Work out the finished part from the listing and answer in its coordinate system (mm). A direction names the side the tool comes from. Coordinates: 2 decimals unless noted, no trailing zeros. Write each loop counter-clockwise with the first axis right and the second up, starting at its lowest first coordinate (ties: lowest second). Pieces come first, ordered by that corner, then holes. Notation, with made-up numbers: (-6.5, 84) - (17.5, 84) arc R29 cw to (17.5, 112) - close; hole circle Ø3 at (75, 37). An arc over 180 degrees is marked (long way). Use one line per item in the form item = value. Start each with the question number.
Item 1: A cutting plane is placed at B-B (x = -5.5). Write down the section's boundary in (y, z), then the cut area to 3 significant figures.
Item 2: A cutting plane is placed at C-C (z = 4). Write down the section's boundary in (x, y) (3 decimals).
Item 3: For faces 4 (the cylindrical face through (-3.971, -3.045, 0.739)), 5 (the flat face through (-4.7, 1.25, -11.6)), 6 (the flat face through (-5.1, 1, -12)), 7 (the flat face through (5.1, 1, -12)), 8 (the flat face through (0, -4.4, 0)), determine the directions among +Z, -Z, +X, -X, +Y, -Y from which every point of the face is accessible in a straight line to the end or side of a thin tool.
Item 4: A cutting plane is placed at A-A (z = -7). Write down the section's boundary in (x, y).
Item 5: Consider probe 1 along Z at (x, y) = (-1.25, 2); probe 2 along Z at (x, y) = (-5, -2.5); probe 3 along Y at (x, z) = (5.25, -7). Determine where each line is inside the solid, lowest interval first.
Item 6: Determine the mould class of faces 1 (the cylindrical face through (0.01, -0.95, -14.65)), 2 (the flat face through (4.7, -1.25, -11.7)), 3 (the cylindrical face through (-0.01, 0.64, -11.82)) for opening direction Z: released by +Z, released by -Z, zero draft, split by the parting line, or undercut.
Item 7: Given pin 1 (0.5 mm diameter, centred on x = 0, y = -4.5, fed in from -Z); pin 2 (4 mm diameter, centred on x = 4.5, y = -1.5, fed in from -Z); pin 3 (2 mm diameter, centred on y = 0.5, z = -12, fed in from +X); pin 4 (1.2 mm diameter, centred on y = 1, z = 5.5, fed in from +X), each flat-ended and moving along its own axis, determine where each tip first touches the part or whether it passes through.
from build123d import *

# Parameters (mm, degrees)
SKETCH2_W           = 13.0048
SKETCH2_H           = 7.8994
BOSS_EXTRUDE1_DEPTH = 9.4234
BOSS_EXTRUDE2_START = 4.7
SKETCH5_R           = 0.95
BOSS_EXTRUDE2_DEPTH = 0.4
LPATTERN1_COUNT     = 3
LPATTERN1_PITCH     = 4.7
SKETCH6_R           = 5.0038
BOSS_EXTRUDE3_DEPTH = 1.4986
BOSS_EXTRUDE5_DEPTH = 7.493


with BuildPart() as part:
    # Sketch2 → Boss-Extrude1 (new body)
    with BuildSketch(Plane.XY):
        Rectangle(SKETCH2_W, SKETCH2_H)
    extrude(amount=-BOSS_EXTRUDE1_DEPTH)

    # Sketch5 → Boss-Extrude2 (add, symmetric)
    with BuildSketch(Plane(origin=(0, 0, 0), x_dir=(0, 0, -1), z_dir=(1, 0, 0)).offset(BOSS_EXTRUDE2_START)):
        with BuildLine():
            ThreePointArc((13.9352, 1.25), (14.642306781, 0.957106781), (14.9352, 0.25))
            Line((14.9352, 0.25), (14.9352, -0.25))
            ThreePointArc((14.9352, -0.25), (14.642306781, -0.957106781), (13.9352, -1.25))
            Line((13.9352, -1.25), (9.4234, -1.25))
            Line((9.4234, -1.25), (9.4234, 1.25))
            Line((9.4234, 1.25), (13.9352, 1.25))
        make_face()
        with Locations((12.5234, 0)):
            Circle(SKETCH5_R, mode=Mode.SUBTRACT)
    boss_extrude2 = extrude(amount=BOSS_EXTRUDE2_DEPTH, both=True)

    # LPattern1: Boss-Extrude2 ×3
    with Locations(*[(-i * LPATTERN1_PITCH, 0, 0) for i in range(1, LPATTERN1_COUNT)]):
        add(boss_extrude2)

    # Sketch6 → Boss-Extrude3 (add)
    with BuildSketch(Plane.XY):
        Circle(SKETCH6_R)
    extrude(amount=BOSS_EXTRUDE3_DEPTH)

    # Sketch7 → Boss-Extrude5 (add)
    with BuildSketch(Plane.XY.offset(1.4986)):
        with BuildLine():
            Line((2.4892, -1.970915615), (2.4892, 1.970915615))
            ThreePointArc((2.4892, 1.970915615), (-3.175, 0), (2.4892, -1.970915615))
        make_face()
    extrude(amount=BOSS_EXTRUDE5_DEPTH)

    # Sketch8 → Revolve1 (revolve)
    with BuildSketch(Plane(origin=(0, 0, 0), x_dir=(1, 0, 0), z_dir=(0, 1, 0))):
        with BuildLine():
            Line((-3.138374402, -19.147892103), (0, -4.9916))
            Line((0, -4.9916), (-1.363885522, -4.689233859))
            Line((-1.363885522, -4.689233859), (-4.199893783, -17.481640441))
            ThreePointArc((-4.199893783, -17.481640441), (-4.014226111, -18.534614134), (-3.138374402, -19.147892103))
        make_face()
    revolve(axis=Axis((-3.138374402, 0, 19.147892103), (0.216439614, 0, -0.976296007)))


solid = part.part
Answer:
q1.outline = (-3.95, -9.42) - (3.95, -9.42) - (3.95, 0) - (-3.95, 0) - close
q1.area = 74.4 mm²
q2.outline = (2.489, -1.971) - (2.489, 1.971) arc R3.175 ccw (long way) to start
q3.face_4 = +Z
q3.face_5 = -Z, +X, -X, +Y
q3.face_6 = -Z, -X, +Y, -Y
q3.face_7 = -Z, +X, +Y, -Y
q3.face_8 = -Z, +X, -X, -Y
q4.outline = (-6.5, -3.95) - (6.5, -3.95) - (6.5, 3.95) - (-6.5, 3.95) - close
q5.probe_1 = -9.42 to 8.99
q5.probe_2 = -9.42 to 0
q5.probe_3 = -3.95 to 3.95
q6.face_1 = released by -Z
q6.face_2 = zero draft
q6.face_3 = undercut
q7.pin_1 = 0
q7.pin_2 = -14.94
q7.pin_3 = 5.1
q7.pin_4 = 2.49
